Verification items for the finished model (mm, model axes). A direction names the side the tool comes from. Round coordinates to 2 decimals unless told otherwise and drop trailing zeros. Order: outer loops, then holes, each group sorted by start corner. A loop starts at its lowest first (then second) coordinate and runs counter-clockwise, first axis right, second up. Notation, with made-up numbers: (6.5, 0) -> (30.5, 0) arc R30 cw to (30.5, 32) -> close; hole circle Ø2 at (6.25, -37.5). An arc over 180 degrees is marked (long way). Return JSON: item names as keys, results as strings. Group by question number.
1) Section check B-B on z = 36.5. Enter the section's corners in (x, y).
2) Section check D-D on y = 43. State how many separate pieces and enclosed holes the cut face has, plus the area to 3 significant figures.
3) Draft check along X on faces 3 (the flat face through (22, 139, 28)), 4 (the flat face through (150, 70, 25)), 5 (the flat face through (74, 72, 0)). Enter one of: pulls with the +X half, pulls with the -X half, needs draft (parallel to the pull), parting line crosses it, or undercut.
4) Scan lines: L1, parallel to X at y = 47, z = 12.5; L2, parallel to X at y = 104, z = 2; L3, parallel to Y at x = 92, z = 2. Record each from-to range of solid material in increasing order.
5) Tool access check on faces 1 (the cylindrical face through (19.91, 96.45, 2.54)), 2 (the flat face through (128, 3, 28)). Record the directions out of +Z, -Z, +X, -X, +Y, -Y that give a thin tool (end or side, any length) a straight path to the whole face; none if there is none.
6) Section check C-C on y = 15. Enter the section's corners in (x, z), plus the area to 3 significant figures.
7) Depth check by flat-ended pin: pin 1 (9.5 mm diameter, centred on x = 121.5, y = 91, fed in from +Z); pin 2 (8 mm diameter, centred on x = 17.5, z = 36, fed in from -Y). Enter the tip coordinate at first touch or a pass-through.
8) Section check A-A on x = 57.25. Enter the section's corners in (y, z), plus the area to 3 significant figures.
```python
from build123d import *

# Parameters (mm, degrees)
SKETCH_W        = 150
SKETCH_H        = 142
PAD_DEPTH       = 50
SKETCH001_W     = 31.5
SKETCH001_H     = 136
POCKET_DEPTH    = 45
SKETCH002_R     = 8.5
SKETCH002_R_2   = 11
POCKET001_DEPTH = 5


with BuildPart() as part:
    # Sketch → Pad (new body)
    with BuildSketch(Plane.XY):
        with Locations((75, 71)):
            Rectangle(SKETCH_W, SKETCH_H)
    extrude(amount=PAD_DEPTH)

    # Sketch001 → Pocket (cut)
    with BuildSketch(Plane.XY.offset(50)):
        with Locations((21.75, 71)):
            Rectangle(SKETCH001_W, SKETCH001_H)
        with Locations((57.25, 71)):
            Rectangle(SKETCH001_W, SKETCH001_H)
        with Locations((92.75, 71)):
            Rectangle(SKETCH001_W, SKETCH001_H)
        with Locations((128.25, 71)):
            Rectangle(SKETCH001_W, SKETCH001_H)
    extrude(amount=-POCKET_DEPTH, mode=Mode.SUBTRACT)

    # Sketch002 → Pocket001 (cut)
    with BuildSketch(Plane.XY.offset(5)):
        with Locations((21.75, 37.25)):
            Circle(SKETCH002_R)
        with Locations((21.75, 71)):
            Circle(SKETCH002_R_2)
        with Locations((21.75, 104.75)):
            Circle(SKETCH002_R)
        with Locations((57.25, 37.25)):
            Circle(SKETCH002_R)
        with Locations((57.25, 71)):
            Circle(SKETCH002_R_2)
        with Locations((57.25, 104.75)):
            Circle(SKETCH002_R)
        with Locations((92.75, 37.25)):
            Circle(SKETCH002_R)
        with Locations((92.75, 71)):
            Circle(SKETCH002_R_2)
        with Locations((92.75, 104.75)):
            Circle(SKETCH002_R)
        with Locations((128.25, 37.25)):
            Circle(SKETCH002_R)
        with Locations((128.25, 71)):
            Circle(SKETCH002_R_2)
        with Locations((128.25, 104.75)):
            Circle(SKETCH002_R)
    extrude(amount=-POCKET001_DEPTH, mode=Mode.SUBTRACT)


solid = part.part
```
Check result:
{
 "1": {"outline": "(0, 0) -> (150, 0) -> (150, 142) -> (0, 142) -> close; hole (6, 3) -> (37.5, 3) -> (37.5, 139) -> (6, 139) -> close; hole (41.5, 3) -> (73, 3) -> (73, 139) -> (41.5, 139) -> close; hole (77, 3) -> (108.5, 3) -> (108.5, 139) -> (77, 139) -> close; hole (112.5, 3) -> (144, 3) -> (144, 139) -> (112.5, 139) -> close"},
 "2": {"separate pieces": "5", "enclosed holes": "0", "area": "1,580 mm^2"},
 "3": {"face 3": "undercut", "face 4": "pulls with the +X half", "face 5": "needs draft"},
 "4": {"L1": "0 to 6, 37.5 to 41.5, 73 to 77, 108.5 to 112.5, 144 to 150", "L2": "0 to 13.28, 30.22 to 48.78, 65.72 to 84.28, 101.22 to 119.78, 136.72 to 150", "L3": "0 to 28.78, 45.72 to 60.03, 81.97 to 96.28, 113.22 to 142"},
 "5": {"face 1": "+Z, -Z", "face 2": "+Z"},
 "6": {"outline": "(0, 0) -> (150, 0) -> (150, 50) -> (144, 50) -> (144, 5) -> (112.5, 5) -> (112.5, 50) -> (108.5, 50) -> (108.5, 5) -> (77, 5) -> (77, 50) -> (73, 50) -> (73, 5) -> (41.5, 5) -> (41.5, 50) -> (37.5, 50) -> (37.5, 5) -> (6, 5) -> (6, 50) -> (0, 50) -> close", "area": "1,830 mm^2"},
 "7": {"pin 1": "z = 5", "pin 2": "y = 0"},
 "8": {"outline": "(0, 0) -> (28.75, 0) -> (28.75, 5) -> (3, 5) -> (3, 50) -> (0, 50) -> close; (45.75, 0) -> (60, 0) -> (60, 5) -> (45.75, 5) -> close; (82, 0) -> (96.25, 0) -> (96.25, 5) -> (82, 5) -> close; (113.25, 0) -> (142, 0) -> (142, 50) -> (139, 50) -> (139, 5) -> (113.25, 5) -> close", "area": "700 mm^2"}
}
